The model under review builds one solid part; all positions refer to its coordinate system, in mm. A direction names the side the tool comes from. Give positions to 0.01 mm unless a question says otherwise; leave off trailing zeros. Loops run counter-clockwise (first coordinate to the right, second up) from the corner with the lowest first, then second, coordinate; pieces in that order, holes last. Notation, with made-up numbers: M 49.25,-7 L 86.25,-7 A26 ccw 86.25,30 Z; hole C -19,36 d3. An arc over 180 degrees is marked long. Put each result on its own line as item: value. Start each with the question number.
Autodesk Inventor part; units mm, degrees
ref_plane "YZ Plane" through (0, 0, 0) normal (1, 0, 0) x (0, 1, 0)
ref_plane "XZ Plane" through (0, 0, 0) normal (0, 1, 0) x (-1, 0, 0)
ref_plane "XY Plane" through (0, 0, 0) normal (0, 0, 1) x (1, 0, 0)
sketch "スケッチ1" plane through (0, 0, 0) normal (0, 0, 1) x (1, 0, 0)
  line L0 (130, 25) -> (130, 30)
  line L1 (130, 30) -> (-10, 30)
  line L2 (-10, 30) -> (-10, 25)
  line L3 (60, 30) -> (60, 0) construction
  line L4 (85, 0) -> (85, 5)
  line L5 (85, 5) -> (35, 5)
  line L6 (35, 5) -> (35, 0)
  line L7 (30, 0) -> (35, 0)
  line L8 (85, 0) -> (90, 0)
  line L9 (30, 0) -> (30, 25)
  line L10 (30, 25) -> (-10, 25)
  line L11 (90, 0) -> (90, 25)
  line L12 (90, 25) -> (130, 25)
  dimension "d2" = 50
  dimension "d4" = 5
  dimension "d5" = 5
  dimension "d6" = 5
  dimension "d7" = 140
  dimension "d8" = 30
extrude "押し出し1" add sketch "スケッチ1" along normal blind 10
sketch "スケッチ2" plane through (0, 0, 0) normal (0, 0, -1) x (-1, 0, 0)
  line L0 (-85, 10) -> (-35, 10)
  line L1 (-35, 10) -> (-35, 25)
  line L2 (-35, 25) -> (-85, 25)
  line L3 (-85, 25) -> (-85, 10)
  line L4 (-90, 0) -> (-90, 25)
  line L5 (-85, 0) -> (-90, 0)
  line L6 (-85, 5) -> (-85, 0)
  line L7 (-35, 5) -> (-85, 5)
  line L8 (-35, 0) -> (-35, 5)
  line L9 (-30, 0) -> (-35, 0)
  line L10 (-30, 25) -> (-30, 0)
  line L11 (10, 25) -> (-30, 25)
  line L12 (10, 30) -> (10, 25)
  line L13 (-130, 30) -> (10, 30)
  line L14 (-130, 25) -> (-130, 30)
  line L15 (-90, 25) -> (-130, 25)
  line L16 (-130, 30) -> (10, 30)
  line L17 (-60, 30) -> (-60, 5) construction
  line L18 (-35, 5) -> (-85, 5)
  point P0 (0, 0)
  dimension "d11" = 5
  dimension "d12" = 5
  dimension "d13" = 50
extrude "押し出し2" cut sketch "スケッチ2" against normal through all contours L3 L2 L1 L0
fillet "フィレット1" radius 1 4 edges at (85, 25, 5) (35, 25, 5) (35, 10, 5) (85, 10, 5)
properties part number "waist1." material "アルミニウム 6061"
Item 1: Consider section D-D, the plane x = 18. Write out the cut boundary in (y, z).
Item 2: To check wall thickness, follow L1, parallel to X at y = 11.5, z = 8; L2, parallel to Y at x = 78.5, z = 2.5; L3, parallel to Y at x = 109, z = 7.75. State the ranges of each line that lie inside material, in increasing order. Write a range as [from, to].
Item 3: Tool access review of faces 4 (the flat face through (85, 2, 5)), 5 (the flat face through (90, 12, 5)), 6 (the flat face through (60, 10, 5)): name each direction out of +Z, -Z, +X, -X, +Y, -Y from which nothing blocks a thin tool from reaching the whole face with its end or side.
Item 4: Draft analysis for pull direction X (two halves, no side actions). For faces 1 (the flat face through (10, 25, 5)), 2 (the flat face through (60, 25, 5)), 3 (the flat face through (30, 12, 5)), state which applies: +X half, -X half, draft (parallel to the pull), parting line (faces both ways), or undercut.
Item 5: Consider section B-B, the plane z = 6. Write out the cut boundary in (x, y), plus the area to 3 significant figures.
Item 6: Clearance check with flat-ended pins moving along their axes: pin 1 Ø5 at (y, z) = (9.5, 6) entering from -X; pin 2 Ø1.5 at (y, z) = (1.5, 4) entering from +X; pin 3 Ø12 at (x, y) = (99, 13) entering from -Z; pin 4 Ø5 at (x, z) = (61.5, 5) entering from -Y. State where each tip first meets the part, or that it passes through.
Item 7: Consider section A-A, the plane x = 48.5. Write out the cut boundary in (y, z), plus the area to 3 significant figures.
Item 8: Consider section C-C, the plane y = 6.75. Write out the cut boundary in (x, z), plus the area to 3 significant figures.
Report:
1. outline: M 25,0 L 30,0 L 30,10 L 25,10 Z
2. L1: [30, 35], [85, 90]
2. L2: [5, 10], [25, 30]
2. L3: [25, 30]
3. face 4: +Z, -Z, -Y
3. face 5: +Z, -Z, +X, -Y
3. face 6: +Z, -Z
4. face 1: draft
4. face 2: undercut
4. face 3: -X half
5. outline: M -10,25 L 30,25 L 30,0 L 35,0 L 35,5 L 85,5 L 85,0 L 90,0 L 90,25 L 130,25 L 130,30 L -10,30 Z; hole M 35,11 A1 ccw 36,10 L 84,10 A1 ccw 85,11 L 85,24 A1 ccw 84,25 L 36,25 A1 ccw 35,24 Z
5. area: 1,200 mm²
6. pin 1: x = 30
6. pin 2: x = 90
6. pin 3: through
6. pin 4: y = 5
7. outline: M 5,0 L 10,0 L 10,10 L 5,10 Z; M 25,0 L 30,0 L 30,10 L 25,10 Z
7. area: 100 mm²
8. outline: M 30,0 L 90,0 L 90,10 L 30,10 Z
8. area: 600 mm²
